from build123d import *

# Parameters (mm, degrees)
SKETCH_W            = 1200
SKETCH_H            = 144
SKETCH_W_2          = 382.5
SKETCH_H_2          = 78
PAD_DEPTH           = 400
PAD_DEPTH_BACK      = 400
SKETCH001_W         = 100
SKETCH001_H         = 227.5
SKETCH001_W_2       = 22
SKETCH001_H_2       = 40
POCKET_DEPTH        = 1200
MIRROREDSKETCH_W    = 100
MIRROREDSKETCH_H    = 227.5
MIRROREDSKETCH_W_2  = 22
MIRROREDSKETCH_H_2  = 40
POCKET001_DEPTH     = 1200
SKETCH002_W         = 382.5
SKETCH002_H         = 100
POCKET002_DEPTH     = 800
MIRROREDSKETCH002_W = 382.5
MIRROREDSKETCH002_H = 100
POCKET003_DEPTH     = 800


with BuildPart() as part:
    # Sketch → Pad (new body, two sides)
    with BuildSketch(Plane.YZ) as pad_sk:
        Rectangle(SKETCH_W, SKETCH_H)
        with Locations((-263.75, -11)):
            Rectangle(SKETCH_W_2, SKETCH_H_2, mode=Mode.SUBTRACT)
        with Locations((263.75, -11)):
            Rectangle(SKETCH_W_2, SKETCH_H_2, mode=Mode.SUBTRACT)
    extrude(amount=PAD_DEPTH)
    extrude(pad_sk.sketch, amount=-PAD_DEPTH_BACK)

    # Sketch001 (on Face4 of Pad) → Pocket (cut)
    with BuildSketch(Plane(origin=(0, -600, 0), x_dir=(0, 0, -1), z_dir=(0, -1, 0))):
        with Locations((22, 186.25)):
            Rectangle(SKETCH001_W, SKETCH001_H)
        with Locations((-61, 92.5)):
            Rectangle(SKETCH001_W_2, SKETCH001_H_2)
        with Locations((-61, 232.5)):
            Rectangle(SKETCH001_W_2, SKETCH001_H_2)
    extrude(amount=-POCKET_DEPTH, mode=Mode.SUBTRACT)

    # MirroredSketch → Pocket001 (cut)
    with BuildSketch(Plane(origin=(0, -600, 0), x_dir=(0, 0, -1), z_dir=(0, -1, 0))):
        with Locations((22, -186.25)):
            Rectangle(MIRROREDSKETCH_W, MIRROREDSKETCH_H)
        with Locations((-61, -92.5)):
            Rectangle(MIRROREDSKETCH_W_2, MIRROREDSKETCH_H_2)
        with Locations((-61, -232.5)):
            Rectangle(MIRROREDSKETCH_W_2, MIRROREDSKETCH_H_2)
    extrude(amount=-POCKET001_DEPTH, mode=Mode.SUBTRACT)

    # Sketch002 (on Face31 of Pocket001) → Pocket002 (cut)
    with BuildSketch(Plane.YZ.offset(400)):
        with Locations((-263.75, 0)):
            Rectangle(SKETCH002_W, SKETCH002_H)
    extrude(amount=-POCKET002_DEPTH, mode=Mode.SUBTRACT)

    # MirroredSketch002 → Pocket003 (cut)
    with BuildSketch(Plane.YZ.offset(400)):
        with Locations((263.75, 0)):
            Rectangle(MIRROREDSKETCH002_W, MIRROREDSKETCH002_H)
    extrude(amount=-POCKET003_DEPTH, mode=Mode.SUBTRACT)


solid = part.part
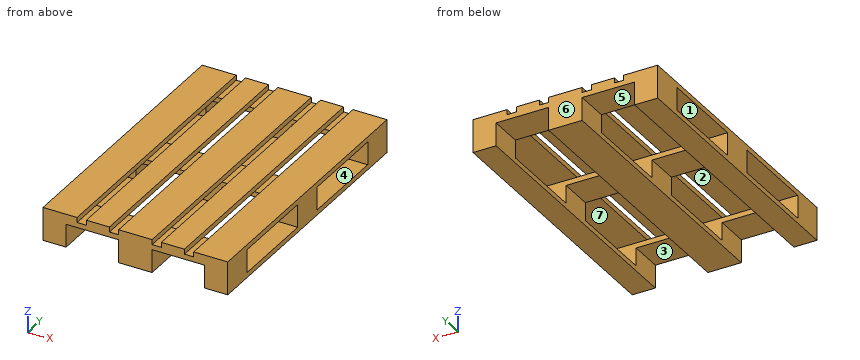
Work out the finished part from the listing and answer in its coordinate system (mm). Face numbers are marked on the shaded views. A direction names the side the tool comes from. Round coordinates to 2 decimals unless told otherwise and drop trailing zeros. Write each loop counter-clockwise with the first axis right and the second up, starting at its lowest first coordinate (ties: lowest second). Pieces come first, ordered by that corner, then holes. Notation, with made-up numbers: (-9.5, 53) -> (15.5, 53) arc R27 ccw to (15.5, 92) -> close; hole circle Ø11 at (72, 33). An arc over 180 degrees is marked (long way). Answer as CSV lines item,"result". Start each with the question number.
(1) The part is cut by section C-C, the plane y = 489. Give the vertices of the cut face in (x, z).
(2) The part is cut by section B-B, the plane x = 85. Give the vertices of the cut face in (y, z), then the cut area to 3 significant figures.
(3) Find the intervals of material crossed by probe 1 along X at (y, z) = (425, -54.5); probe 2 along Y at (x, z) = (74.5, 36.5); probe 3 along X at (y, z) = (420, 64), in increasing order.
(4) This flat-tipped pin is pushed along its axis until it touches: pin 1 (12 mm diameter, centred on x = 230, y = -9, fed in from +Z). Where does it stop, or does it pass through?
(5) The mould has two halves that part along Z. Classify the marked faces 4, 5, 6 and 7: +Z half, -Z half, draft (parallel to the pull), parting line (faces both ways), or undercut.
(6) A tool of negligible diameter and unlimited length cuts with its end or side. For the marked faces 1, 2 and 3, from which of +Z, -Z, +X, -X, +Y, -Y can it reach the whole face along a straight path? Write none if from no direction.
(7) The part is cut by section A-A, the plane y = -299.5. Give the number of separate pieces and of enclosed holes in the cut face, then the cut area to 3 significant figures.
Output values:
1,outline,"(-400, -72) -> (-300, -72) -> (-300, 28) -> (-72.5, 28) -> (-72.5, -72) -> (72.5, -72) -> (72.5, 28) -> (300, 28) -> (300, -72) -> (400, -72) -> (400, 72) -> (252.5, 72) -> (252.5, 50) -> (212.5, 50) -> (212.5, 72) -> (112.5, 72) -> (112.5, 50) -> (72.5, 50) -> (72.5, 72) -> (-72.5, 72) -> (-72.5, 50) -> (-112.5, 50) -> (-112.5, 72) -> (-212.5, 72) -> (-212.5, 50) -> (-252.5, 50) -> (-252.5, 72) -> (-400, 72) -> close"
2,outline,"(-600, 28) -> (-455, 28) -> (-455, 50) -> (-600, 50) -> close; (-72.5, 28) -> (72.5, 28) -> (72.5, 50) -> (-72.5, 50) -> close; (455, 28) -> (600, 28) -> (600, 50) -> (455, 50) -> close"
2,area,"9,570 mm²"
3,probe 1,"x = -400 to -300, -72.5 to 72.5, 300 to 400"
3,probe 2,"y = -600 to -455, -72.5 to 72.5, 455 to 600"
3,probe 3,"x = -400 to -252.5, -212.5 to -112.5, -72.5 to 72.5, 112.5 to 212.5, 252.5 to 400"
4,pin 1,"stops at z = 50"
5,face 4,"undercut"
5,face 5,"-Z half"
5,face 6,"draft"
5,face 7,"undercut"
6,face 1,"+X, -X"
6,face 2,"-Z, +X, -X"
6,face 3,"-Z, +Y, -Y"
7,separate pieces,"8"
7,enclosed holes,"0"
7,area,"21,700 mm²"
